Verification items for the finished model (mm, model axes). Face numbers are marked on the shaded views. A direction names the side the tool comes from. Coordinates: 2 decimals unless noted, no trailing zeros. Write each loop counter-clockwise with the first axis right and the second up, starting at its lowest first coordinate (ties: lowest second). Pieces come first, ordered by that corner, then holes. Notation, with made-up numbers: (8, 48) - (61, 48) arc R21 cw to (61, 60) - close; hole circle Ø5 at (4.5, 48.5). An arc over 180 degrees is marked (long way). Use CSV: the item, a comma, the result in double quotes. Start each with the question number.
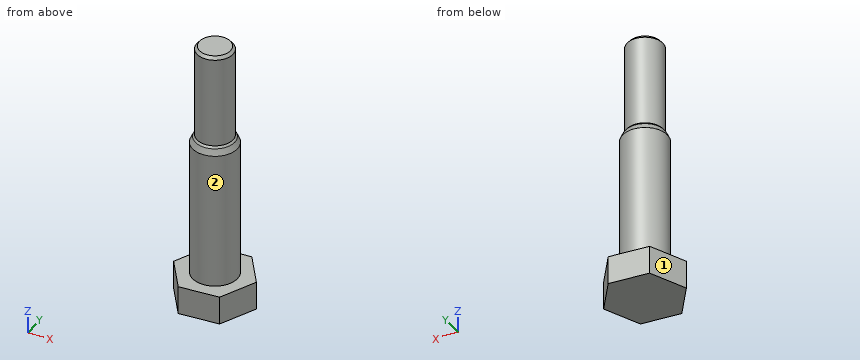
```python
from build123d import *

# Parameters (mm, degrees)
SKETCH_1_R       = 15
EXTRUDE_1_DEPTH  = 111
EXTRUDE_2_DEPTH  = 19
SKETCH_7_R       = 15
EXTRUDE_4_DEPTH  = 4
EXTRUDE_4_TAPER  = 25
SKETCH_22_R      = 12
EXTRUDE_22_DEPTH = 62
SKETCH_23_R      = 13.134769367
EXTRUDE_24_DEPTH = 2
EXTRUDE_24_TAPER = 40
SKETCH_24_R      = 12
EXTRUDE_25_DEPTH = 2
EXTRUDE_25_TAPER = 40


with BuildPart() as part:
    # 草图1 → 拉伸1 (new body)
    with BuildSketch(Plane.XY):
        Circle(SKETCH_1_R)
    extrude(amount=EXTRUDE_1_DEPTH)

    # 草图2 → 拉伸2 (add)
    with BuildSketch(Plane.XY):
        Polygon((14.770690633, -22.071702054), (26.5, 1.755942292), (11.729309367, 23.827644346), (-14.770690633, 22.071702054), (-26.5, -1.755942292), (-11.729309367, -23.827644346), align=None)
    extrude(amount=EXTRUDE_2_DEPTH)

    # 草图7 → 拉伸4 (add)
    with BuildSketch(Plane.XY.offset(111)):
        Circle(SKETCH_7_R)
    extrude(amount=EXTRUDE_4_DEPTH, taper=EXTRUDE_4_TAPER)

    # 草图22 → 拉伸22 (add)
    with BuildSketch(Plane.XY.offset(115)):
        Circle(SKETCH_22_R)
    extrude(amount=EXTRUDE_22_DEPTH)

    # 草图23 → 拉伸24 (add)
    with BuildSketch(Plane.XY.offset(115)):
        Circle(SKETCH_23_R)
    extrude(amount=EXTRUDE_24_DEPTH, taper=EXTRUDE_24_TAPER)

    # 草图24 → 拉伸25 (add)
    with BuildSketch(Plane.XY.offset(177)):
        Circle(SKETCH_24_R)
    extrude(amount=EXTRUDE_25_DEPTH, taper=EXTRUDE_25_TAPER)


solid = part.part
```
Q1. Cross-section at A-A (y = 0). Record the cut outline in (x, z), plus the area to 3 significant figures.
Q2. Cross-section at B-B (z = 151). Record the cut outline in (x, y).
Q3. Scan lines: line 1 along Z through (x, y) = (9, -18.5); line 2 along X through (y, z) = (-0.5, 46.5); line 3 along Y through (x, z) = (-0.5, 122). Record each from-to range of solid material in increasing order. Write a range as from..to.
Q4. Cross-section at C-C (x = 0). Record the cut outline in (y, z), plus the area to 3 significant figures.
Q5. Cross-section at D-D (z = 94). Record the cut outline in (x, y).
Q6. Tool access check on the marked faces 1 and 2. Record the directions out of +Z, -Z, +X, -X, +Y, -Y that give a thin tool (end or side, any length) a straight path to the whole face; none if there is none.
Q7. Gauge pin test, flat ends, axial feed: pin 1 (1 mm diameter, centred on x = -1.5, y = -10.5, fed in from -Z); pin 2 (2 mm diameter, centred on x = 9.5, z = 75.5, fed in from -Y); pin 3 (5 mm diameter, centred on x = 19, z = 24, fed in from +Y); pin 4 (1.5 mm diameter, centred on y = 4, z = 146.5, fed in from +X). Record the tip position at first contact, or that the pin passes through.
Reply:
1,outline,"(-25.64, 0) - (25.64, 0) - (25.64, 19) - (15, 19) - (15, 111) - (13.13, 115) - (12, 116.35) - (12, 177) - (10.32, 179) - (-10.32, 179) - (-12, 177) - (-12, 116.35) - (-13.13, 115) - (-15, 111) - (-15, 19) - (-25.64, 19) - close"
1,area,"5,380 mm^2"
2,outline,"circle Ø24 at (0, 0)"
3,line 1,"0..19"
3,line 2,"-14.99..14.99"
3,line 3,"-11.99..11.99"
4,outline,"(-23.05, 0) - (23.05, 0) - (23.05, 19) - (15, 19) - (15, 111) - (13.13, 115) - (12, 116.35) - (12, 177) - (10.32, 179) - (-10.32, 179) - (-12, 177) - (-12, 116.35) - (-13.13, 115) - (-15, 111) - (-15, 19) - (-23.05, 19) - close"
4,area,"5,280 mm^2"
5,outline,"circle Ø30 at (0, 0)"
6,face 1,"+Z, -Z, -X, +Y"
6,face 2,"+Z"
7,pin 1,"z = 0"
7,pin 2,"y = -12.36"
7,pin 3,"through"
7,pin 4,"x = 11.55"
